CAD build for the part. Positions are in the model's coordinates, mm. Coordinates: 2 decimals unless noted, no trailing zeros. Loops run counter-clockwise (first coordinate to the right, second up) from the corner with the lowest first, then second, coordinate; pieces in that order, holes last. Notation, with made-up numbers: (58, 2.25) - (112, 2.25) arc R19 cw to (112, 14.25) - close; hole circle Ø11 at (-10, 79.25). An arc over 180 degrees is marked (long way). Put each result on its own line as item: value.
```python
from build123d import *

# Parameters (mm, degrees)
SKETCH1_W           = 15
SKETCH1_H           = 465
BOSS_EXTRUDE1_DEPTH = 20
SKETCH2_W           = 12.5
SKETCH2_H           = 465
CUT_EXTRUDE1_DEPTH  = 5
SKETCH4_W           = 465
SKETCH4_H           = 20
BOSS_EXTRUDE3_DEPTH = 27.5


with BuildPart() as part:
    # Sketch1 → Boss-Extrude1 (new body)
    with BuildSketch(Plane(origin=(0, 0, 0), x_dir=(1, 0, 0), z_dir=(0, 1, 0))):
        Rectangle(SKETCH1_W, SKETCH1_H)
    extrude(amount=BOSS_EXTRUDE1_DEPTH)

    # Sketch2 → Cut-Extrude1 (cut)
    with BuildSketch(Plane(origin=(0, 20, 0), x_dir=(1, 0, 0), z_dir=(0, 1, 0))):
        Rectangle(SKETCH2_W, SKETCH2_H)
    extrude(amount=-CUT_EXTRUDE1_DEPTH, mode=Mode.SUBTRACT)

    # Sketch4 → Boss-Extrude3 (add)
    with BuildSketch(Plane.ZY.offset(-7.5)):
        with Locations((0, 10)):
            Rectangle(SKETCH4_W, SKETCH4_H)
    extrude(amount=-BOSS_EXTRUDE3_DEPTH)


solid = part.part
```
Q1. Slice it at A-A, the plane z = -14.5. Give the cut face in (x, y).
Determined:
outline: (-7.5, 0) - (35, 0) - (35, 20) - (6.25, 20) - (6.25, 15) - (-6.25, 15) - (-6.25, 20) - (-7.5, 20) - close
Q2. Wall check: L1, parallel to X at y = 18.75, z = 85.5; L2, parallel to Y at x = -3, z = 152. Give the ranges that are in metal, low to high. Write a range as from..to.
Determined:
L1: -7.5..-6.25, 6.25..35
L2: 0..15
Q3. Slice it at B-B, the plane x = -1. Give the cut face in (y, z).
Determined:
outline: (0, -232.5) - (15, -232.5) - (15, 232.5) - (0, 232.5) - close
Q4. Mould opens along X. For faces 1 (the flat face through (13, 10, 232.5)), 2 (the flat face through (35, 10, -3)), 3 (the flat face through (-7.5, 10, 3)), 4 (the flat face through (0, 15, -3)) say: +X half, -X half, draft (parallel to the pull), parting line (faces both ways), or undercut.
Determined:
face 1: draft
face 2: +X half
face 3: -X half
face 4: undercut
Q5. Pin check, flat tips, straight feed: pin 1 Ø8 at (x, z) = (18, -132.5) entering from -Y; pin 2 Ø6 at (x, z) = (-2, -66) entering from +Y. Stop position of each tip, or through.
Determined:
pin 1: y = 0
pin 2: y = 15
